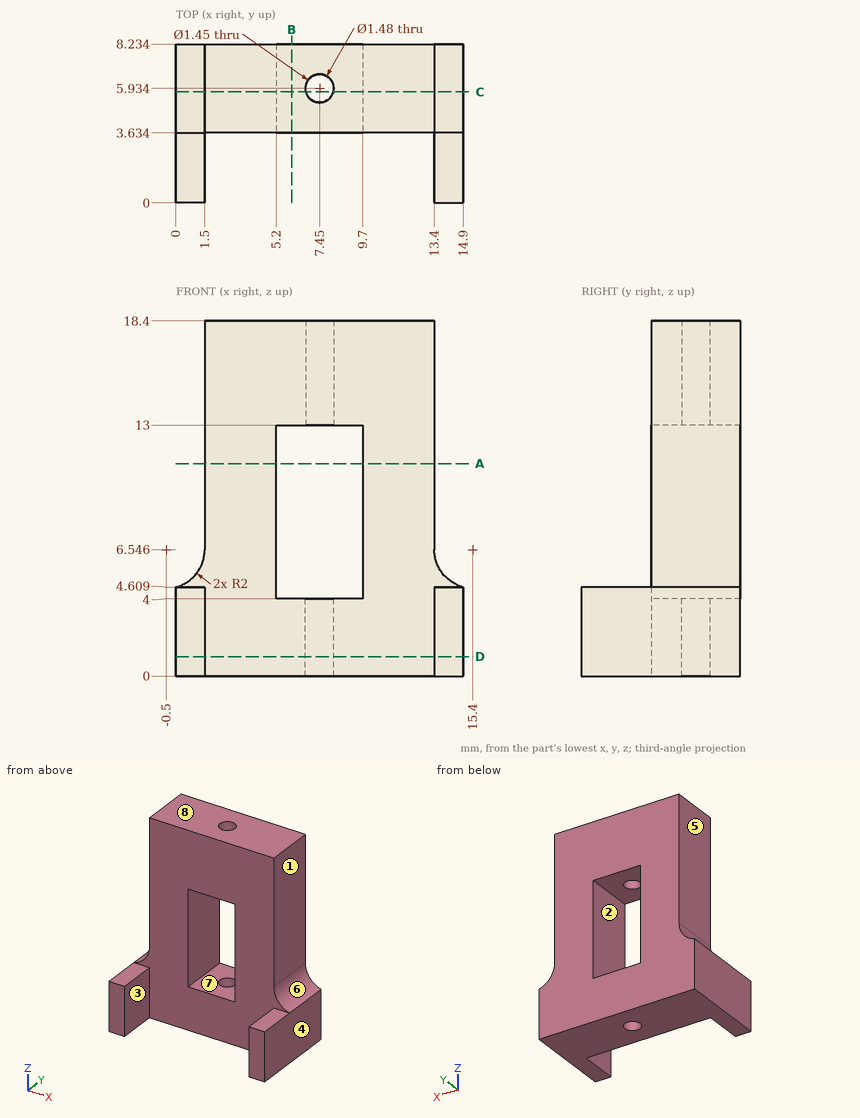
Geometry check sheet. Reference: drawing and pictorial views, mm from the part's lowest x, y, z. A direction names the side the tool comes from. Give positions to 0.01 mm unless a question says otherwise; leave off trailing zeros. Order: outer loops, then holes, each group sorted by start corner. A loop starts at its lowest first (then second) coordinate and runs counter-clockwise, first axis right, second up. Notation, with made-up numbers: (84, 71) - (91, 71) arc R21 ccw to (91, 88) - close; hole circle Ø9 at (-33.5, -24.5). An arc over 180 degrees is marked (long way). Answer as CSV lines item,"result". Start each with the question number.
Item 1: Access from +Z, -Z, +X, -X, +Y, -Y to the whole of each face (thin tool, end or side, straight path). Record for the marked faces 1, 2, 3, 4 and 5.
Item 2: Section check C-C, the plane y = 5.75. Record the boundary of the cut face in (x, z).
Item 3: Mould release check, pull along X, two halves, no side actions. Record for the marked faces 6, 7 and 8: released by +X, released by -X, zero draft, split by the parting line, or undercut.
Item 4: Gauge pin test, flat ends, axial feed: pin 1 (2.5 mm diameter, centred on y = 5.5, z = 8.5, fed in from -X); pin 2 (3 mm diameter, centred on x = 11, z = 12, fed in from -Y); pin 3 (1.4 mm diameter, centred on y = 5.5, z = 8.5, fed in from +X); pin 4 (1.9 mm diameter, centred on x = 7.45, y = 5.93, fed in from +Z). Record the tip position at first contact, or that the pin passes through.
Item 5: Material ranges on L1, parallel to X at y = 6.25, z = 8.5; L2, parallel to Y at x = 7.5, z = 13.25 (1 decimal); L3, parallel to Z at x = 6, y = 6.5, recorded low to high.
Item 6: Section check D-D, the plane z = 1. Record the boundary of the cut face in (x, y).
Item 7: Section check A-A, the plane z = 11. Record the boundary of the cut face in (x, y).
Item 8: Section check B-B, the plane x = 6. Record the boundary of the cut face in (y, z).
Filled in:
1,face 1,"+Z, +X, +Y, -Y"
1,face 2,"+Y, -Y"
1,face 3,"+Z, -Z, -Y"
1,face 4,"+Z, -Z, +X, +Y, -Y"
1,face 5,"+Z, -X, +Y, -Y"
2,outline,"(0, 0) - (6.73, 0) - (6.73, 4) - (5.2, 4) - (5.2, 13) - (6.75, 13) - (6.75, 18.4) - (1.5, 18.4) - (1.5, 6.55) arc R2 cw to (0, 4.61) - close; (8.15, 13) - (9.7, 13) - (9.7, 4) - (8.17, 4) - (8.17, 0) - (14.9, 0) - (14.9, 4.61) arc R2 cw to (13.4, 6.55) - (13.4, 18.4) - (8.15, 18.4) - close"
3,face 6,"released by +X"
3,face 7,"undercut"
3,face 8,"zero draft"
4,pin 1,"x = 1.5"
4,pin 2,"y = 3.63"
4,pin 3,"x = 13.4"
4,pin 4,"z = 18.4"
5,L1,"1.5 to 5.2, 9.7 to 13.4"
5,L2,"3.6 to 5.2, 6.7 to 8.2"
5,L3,"0 to 4, 13 to 18.4"
6,outline,"(0, 0) - (1.5, 0) - (1.5, 3.63) - (13.4, 3.63) - (13.4, 0) - (14.9, 0) - (14.9, 8.23) - (0, 8.23) - close; hole circle Ø1.48 at (7.45, 5.93)"
7,outline,"(1.5, 3.63) - (5.2, 3.63) - (5.2, 8.23) - (1.5, 8.23) - close; (9.7, 3.63) - (13.4, 3.63) - (13.4, 8.23) - (9.7, 8.23) - close"
8,outline,"(3.63, 0) - (8.23, 0) - (8.23, 4) - (3.63, 4) - close; (3.63, 13) - (8.23, 13) - (8.23, 18.4) - (3.63, 18.4) - close"
